Input: part model. Units: mm. Frame: model coordinates. A direction names the side the tool comes from. Round coordinates to 2 decimals unless told otherwise and drop trailing zeros. Order: outer loops, then holes, each group sorted by start corner. A loop starts at its lowest first (then second) coordinate and runs counter-clockwise, first axis right, second up.
Item 1: Cut plane A-A on z = 0. Give the number of separate pieces and of enclosed holes in the cut face, then the cut area to 3 significant figures.
Item 2: Mould query, pull axis X, two halves, no side actions, for faces 3 (the cylindrical face through (22.4, 3, -7.1)), 4 (the cylindrical face through (-0.92, 2.46, -7.04)), 5 (the flat face through (16, 6, 16)). Classes: released by +X, released by -X, zero draft, split by the parting line, or undercut.
Item 3: Cut plane B-B on z = 19. Output: boundary loops of the cut face in (x, y), then the cut area to 3 significant figures.
Item 4: First-contact query: pin 1 (1 mm diameter, centred on x = 12, y = 2, fed in from +Z); pin 2 (1 mm diameter, centred on y = 4, z = -16.5, fed in from -X); pin 3 (7 mm diameter, centred on x = -2.5, z = 0.5, fed in from -Y). Flat tips, straight axial feed; report the tip coordinate or a pass-through.
Item 5: Reachability of faces 1 (the cylindrical face through (-0.228, 1.775, 20.735)), 2 (the cylindrical face through (-4.769, 6.296, 21.477)) from +Z, -Z, +X, -X, +Y, -Y: full face, straight path, thin tool, end or side. Return the list, or none.
Item 6: Line query: L1, parallel to Z at x = 0, y = 0.8; L2, parallel to Z at x = 0, y = 5.7; L3, parallel to Z at x = -17, y = 1.75. Output: solid intervals per line, ascending.
Item 7: Cut plane C-C on x = -19. Output: boundary loops of the cut face in (y, z), then the cut area to 3 significant figures.
```python
from build123d import *

# Parameters (mm, degrees)
SKETCH1_R                = 23.5
SKETCH1_R_2              = 7.1
BOSS_EXTRUDE1_DEPTH      = 6
SKETCH2_R                = 22
SKETCH2_R_2              = 5
BOSS_EXTRUDE2_DEPTH      = 0.6
BOSS_EXTRUDE2_DEPTH_BACK = 1
SKETCH3_R                = 1.75
CUT_EXTRUDE1_DEPTH       = 7.6
CUT_EXTRUDE2_START       = -6.6
SKETCH4_R                = 2.75
SKETCH4_R_2              = 1.75
CUT_EXTRUDE2_DEPTH       = 3
SKETCH5_R                = 1.5
CUT_EXTRUDE3_DEPTH       = 7.6


with BuildPart() as part:
    # Sketch1 → Boss-Extrude1 (new body)
    with BuildSketch(Plane(origin=(0, 0, 0), x_dir=(1, 0, 0), z_dir=(0, 1, 0))):
        Circle(SKETCH1_R)
        Circle(SKETCH1_R_2, mode=Mode.SUBTRACT)
    extrude(amount=BOSS_EXTRUDE1_DEPTH)

    # Sketch2 → Boss-Extrude2 (add, two sides)
    with BuildSketch(Plane(origin=(0, 6, 0), x_dir=(1, 0, 0), z_dir=(0, 1, 0))) as boss_extrude2_sk:
        Circle(SKETCH2_R)
        Circle(SKETCH2_R_2, mode=Mode.SUBTRACT)
    extrude(amount=BOSS_EXTRUDE2_DEPTH)
    extrude(boss_extrude2_sk.sketch, amount=-BOSS_EXTRUDE2_DEPTH_BACK)

    # Sketch3 → Cut-Extrude1 (cut, through all)
    with BuildSketch(Plane.XZ):
        with Locations((0, 19)):
            Circle(SKETCH3_R)
        with Locations((19, 0)):
            Circle(SKETCH3_R)
        with Locations((0, -19)):
            Circle(SKETCH3_R)
        with Locations((-19, 0)):
            Circle(SKETCH3_R)
    extrude(amount=-CUT_EXTRUDE1_DEPTH, mode=Mode.SUBTRACT)

    # Sketch4 → Cut-Extrude2 (cut)
    with BuildSketch(Plane(origin=(0, 0, 0), x_dir=(-1, 0, 0), z_dir=(0, -1, 0)).offset(CUT_EXTRUDE2_START)):
        with Locations((0, 19)):
            Circle(SKETCH4_R)
        with Locations((0, 19)):
            Circle(SKETCH4_R_2, mode=Mode.SUBTRACT)
        with Locations((19, 0)):
            Circle(SKETCH4_R)
        with Locations((19, 0)):
            Circle(SKETCH4_R_2, mode=Mode.SUBTRACT)
        with Locations((-19, 0)):
            Circle(SKETCH4_R)
        with Locations((-19, 0)):
            Circle(SKETCH4_R_2, mode=Mode.SUBTRACT)
        with Locations((0, -19)):
            Circle(SKETCH4_R)
        with Locations((0, -19)):
            Circle(SKETCH4_R_2, mode=Mode.SUBTRACT)
    extrude(amount=CUT_EXTRUDE2_DEPTH, mode=Mode.SUBTRACT)

    # Sketch5 → Cut-Extrude3 (cut, through all)
    with BuildSketch(Plane(origin=(0, 6.6, 0), x_dir=(1, 0, 0), z_dir=(0, 1, 0))):
        with Locations((-6.50561835, 15.705952053)):
            Circle(SKETCH5_R)
        with Locations((6.50561835, 15.705952053)):
            Circle(SKETCH5_R)
        with Locations((15.705952053, 6.50561835)):
            Circle(SKETCH5_R)
        with Locations((15.705952053, -6.50561835)):
            Circle(SKETCH5_R)
        with Locations((6.50561835, -15.705952053)):
            Circle(SKETCH5_R)
        with Locations((-6.50561835, -15.705952053)):
            Circle(SKETCH5_R)
        with Locations((-15.705952053, -6.50561835)):
            Circle(SKETCH5_R)
        with Locations((-15.705952053, 6.50561835)):
            Circle(SKETCH5_R)
    extrude(amount=-CUT_EXTRUDE3_DEPTH, mode=Mode.SUBTRACT)


solid = part.part
```
From the geometry:
1. separate pieces: 4
1. enclosed holes: 0
1. area: 163 mm2
2. face 3: split by the parting line
2. face 4: undercut
2. face 5: zero draft
3. outline: (-13.83, 0) - (-1.75, 0) - (-1.75, 3.6) - (-2.75, 3.6) - (-2.75, 6.6) - (-11.09, 6.6) - (-11.09, 6) - (-13.83, 6) - close; (1.75, 0) - (13.83, 0) - (13.83, 6) - (11.09, 6) - (11.09, 6.6) - (2.75, 6.6) - (2.75, 3.6) - (1.75, 3.6) - close
3. area: 150 mm2
4. pin 1: stops at z = 20.49
4. pin 2: stops at x = -17.21
4. pin 3: stops at y = 5
5. face 1: +Y, -Y
5. face 2: +Y
6. L1: z = -23.5 to -20.75, -17.25 to -7.1, 7.1 to 17.25, 20.75 to 23.5
6. L2: z = -23.5 to -21.75, -16.25 to -5, 5 to 16.25, 21.75 to 23.5
6. L3: z = -16.22 to -7.26, -5.75 to 5.75, 7.26 to 16.22
7. outline: (0, -13.83) - (6, -13.83) - (6, -11.09) - (6.6, -11.09) - (6.6, -2.75) - (3.6, -2.75) - (3.6, -1.75) - (0, -1.75) - close; (0, 1.75) - (3.6, 1.75) - (3.6, 2.75) - (6.6, 2.75) - (6.6, 11.09) - (6, 11.09) - (6, 13.83) - (0, 13.83) - close
7. area: 150 mm2
